```python
from build123d import *

# Parameters (mm, degrees)
EXTRUDE_1_DEPTH = 3
FILLET_1_R      = 1.5


with BuildPart() as part:
    # 草图1 → 凸台-拉伸1 (new body)
    with BuildSketch(Plane.XY):
        with BuildLine():
            Line((100.55, -9.975), (100.55, 9.975))
            Line((100.55, 9.975), (93.45, 9.975))
            ThreePointArc((93.45, 9.975), (92.4, 11.025), (93.45, 12.075))
            Line((93.45, 12.075), (93.45, 14.975))
            Line((93.45, 14.975), (49.05, 14.975))
            Line((49.05, 14.975), (49.05, 12.125))
            ThreePointArc((49.05, 12.125), (49.79246212, 11.81746212), (50.1, 11.075))
            ThreePointArc((50.1, 11.075), (49.79246212, 10.33253788), (49.05, 10.025))
            Line((49.05, 10.025), (45.95, 10.025))
            ThreePointArc((45.95, 10.025), (44.9, 11.075), (45.95, 12.125))
            Line((45.95, 12.125), (45.95, 14.975))
            Line((45.95, 14.975), (1.55, 14.975))
            Line((1.55, 14.975), (1.55, 12.075))
            ThreePointArc((1.55, 12.075), (2.29246212, 11.76746212), (2.6, 11.025))
            ThreePointArc((2.6, 11.025), (2.29246212, 10.28253788), (1.55, 9.975))
            Line((1.55, 9.975), (-5.55, 9.975))
            Line((-5.55, 9.975), (-5.55, -9.975))
            Line((-5.55, -9.975), (1.55, -9.975))
            ThreePointArc((1.55, -9.975), (2.29246212, -10.28253788), (2.6, -11.025))
            ThreePointArc((2.6, -11.025), (2.29246212, -11.76746212), (1.55, -12.075))
            Line((1.55, -12.075), (1.55, -14.975))
            Line((1.55, -14.975), (45.95, -14.975))
            Line((45.95, -14.975), (45.95, -12.125))
            ThreePointArc((45.95, -12.125), (44.9, -11.075), (45.95, -10.025))
            Line((45.95, -10.025), (49.05, -10.025))
            ThreePointArc((49.05, -10.025), (49.79246212, -10.33253788), (50.1, -11.075))
            ThreePointArc((50.1, -11.075), (49.79246212, -11.81746212), (49.05, -12.125))
            Line((49.05, -12.125), (49.05, -14.975))
            Line((49.05, -14.975), (93.45, -14.975))
            Line((93.45, -14.975), (93.45, -12.075))
            ThreePointArc((93.45, -12.075), (92.4, -11.025), (93.45, -9.975))
            Line((93.45, -9.975), (100.55, -9.975))
        make_face()
        with BuildLine():
            ThreePointArc((2.6, -3.075), (2.29246212, -3.81746212), (1.55, -4.125))
            Line((1.55, -4.125), (-1.55, -4.125))
            ThreePointArc((-1.55, -4.125), (-2.6, -3.075), (-1.55, -2.025))
            Line((-1.55, -2.025), (-1.55, 2.025))
            ThreePointArc((-1.55, 2.025), (-2.6, 3.075), (-1.55, 4.125))
            Line((-1.55, 4.125), (1.55, 4.125))
            ThreePointArc((1.55, 4.125), (2.29246212, 3.81746212), (2.6, 3.075))
            ThreePointArc((2.6, 3.075), (2.29246212, 2.33253788), (1.55, 2.025))
            Line((1.55, 2.025), (1.55, -2.025))
            ThreePointArc((1.55, -2.025), (2.29246212, -2.33253788), (2.6, -3.075))
        make_face(mode=Mode.SUBTRACT)
        Polygon((39.221033587, -11.975), (8.278966413, -11.975), (23.75, -1.795569934), align=None, mode=Mode.SUBTRACT)
        Polygon((26.478966413, 0), (41.95, 10.179430066), (41.95, -10.179430066), align=None, mode=Mode.SUBTRACT)
        with BuildLine():
            ThreePointArc((50.1, -3.075), (49.79246212, -3.81746212), (49.05, -4.125))
            Line((49.05, -4.125), (45.95, -4.125))
            ThreePointArc((45.95, -4.125), (44.9, -3.075), (45.95, -2.025))
            Line((45.95, -2.025), (45.95, 2.025))
            ThreePointArc((45.95, 2.025), (44.9, 3.075), (45.95, 4.125))
            Line((45.95, 4.125), (49.05, 4.125))
            ThreePointArc((49.05, 4.125), (49.79246212, 3.81746212), (50.1, 3.075))
            ThreePointArc((50.1, 3.075), (49.79246212, 2.33253788), (49.05, 2.025))
            Line((49.05, 2.025), (49.05, -2.025))
            ThreePointArc((49.05, -2.025), (49.79246212, -2.33253788), (50.1, -3.075))
        make_face(mode=Mode.SUBTRACT)
        Polygon((55.778966413, -11.975), (71.25, -1.795569934), (86.721033587, -11.975), align=None, mode=Mode.SUBTRACT)
        Polygon((53.05, 10.179430066), (68.521033587, 0), (53.05, -10.179430066), align=None, mode=Mode.SUBTRACT)
        with BuildLine():
            ThreePointArc((97.6, -3.075), (97.29246212, -3.81746212), (96.55, -4.125))
            Line((96.55, -4.125), (93.45, -4.125))
            ThreePointArc((93.45, -4.125), (92.4, -3.075), (93.45, -2.025))
            Line((93.45, -2.025), (93.45, 2.025))
            ThreePointArc((93.45, 2.025), (92.4, 3.075), (93.45, 4.125))
            Line((93.45, 4.125), (96.55, 4.125))
            ThreePointArc((96.55, 4.125), (97.29246212, 3.81746212), (97.6, 3.075))
            ThreePointArc((97.6, 3.075), (97.29246212, 2.33253788), (96.55, 2.025))
            Line((96.55, 2.025), (96.55, -2.025))
            ThreePointArc((96.55, -2.025), (97.29246212, -2.33253788), (97.6, -3.075))
        make_face(mode=Mode.SUBTRACT)
        Polygon((21.021033587, 0), (5.55, -10.179430066), (5.55, 10.179430066), align=None, mode=Mode.SUBTRACT)
        Polygon((23.75, 1.795569934), (8.278966413, 11.975), (39.221033587, 11.975), align=None, mode=Mode.SUBTRACT)
        Polygon((55.778966413, 11.975), (86.721033587, 11.975), (71.25, 1.795569934), align=None, mode=Mode.SUBTRACT)
        Polygon((89.45, 10.179430066), (89.45, -10.179430066), (73.978966413, 0), align=None, mode=Mode.SUBTRACT)
    extrude(amount=EXTRUDE_1_DEPTH)

    # 圆角1
    fillet_1_edges = [part.edges().sort_by_distance(p)[0] for p in [
        (55.778966413, 11.975, 1.5),
        (71.25, 1.795569934, 1.5),
        (86.721033587, 11.975, 1.5),
        (8.278966413, -11.975, 1.5),
        (39.221033587, -11.975, 1.5),
        (23.75, -1.795569934, 1.5),
        (41.95, -10.179430066, 1.5),
        (41.95, 10.179430066, 1.5),
        (26.478966413, 0, 1.5),
        (21.021033587, 0, 1.5),
        (5.55, 10.179430066, 1.5),
        (5.55, -10.179430066, 1.5),
        (39.221033587, 11.975, 1.5),
        (8.278966413, 11.975, 1.5),
        (23.75, 1.795569934, 1.5),
        (53.05, -10.179430066, 1.5),
        (68.521033587, 0, 1.5),
        (53.05, 10.179430066, 1.5),
        (86.721033587, -11.975, 1.5),
        (71.25, -1.795569934, 1.5),
        (55.778966413, -11.975, 1.5),
        (73.978966413, 0, 1.5),
        (89.45, -10.179430066, 1.5),
        (89.45, 10.179430066, 1.5),
    ]]
    fillet(fillet_1_edges, radius=FILLET_1_R)


solid = part.part
```
Work out the finished part from the listing and answer in its coordinate system (mm). A direction names the side the tool comes from. Give positions to 0.01 mm unless a question says otherwise; leave off trailing zeros. Write each loop counter-clockwise with the first axis right and the second up, starting at its lowest first coordinate (ties: lowest second). Pieces come first, ordered by that corner, then holes. Notation, with made-up numbers: (-6.75, -35) -> (22.25, -35) arc R24 cw to (22.25, 4) -> close; hole circle Ø7 at (48, 20.5). An arc over 180 degrees is marked (long way). Write item = value, one per line.
Q1. For a pull along X with two mould halves and no side action, classify faces 3 (the flat face through (1.55, -14, 1)), 4 (the flat face through (71, -14.975, 1)), 5 (the cylindrical face through (83.14, -10.93, 1.52)), 6 (the cylindrical face through (27.71, -0.02, 1.52)) as pulls with the +X half, pulls with the -X half, needs draft (parallel to the pull), parting line crosses it, or undercut.
Computed values:
face_3 = pulls with the -X half
face_4 = needs draft
face_5 = undercut
face_6 = undercut
Q2. Consider line 1 along Y through (x, z) = (46, 1.55) (3 decimals); line 2 along Y through (x, z) = (22.5, 1) (3 decimals); line 3 along Y through (x, z) = (30, 2.95) (3 decimals). Determine where each line is inside the solid, lowest interval first.
Computed values:
line_1 = -10.025 to -4.125, 4.125 to 10.025
line_2 = -14.975 to -11.975, -2.618 to 2.618, 11.975 to 14.975
line_3 = -14.975 to -11.975, -5.908 to -2.317, 2.317 to 5.908, 11.975 to 14.975
Q3. A tool of negligible diameter and unlimited length cuts with its end or side. For faces 1 (the cylindrical face through (41.182, 8.706, 1.521)), 2 (the cylindrical face through (92.4, 11, 1.5)), from which of +Z, -Z, +X, -X, +Y, -Y can it reach the whole face along a straight path? Write none if from no direction.
Computed values:
face_1 = +Z, -Z
face_2 = +Z, -Z, +X
Q4. Section B-B on y = -6.5 is taken. Determine the outline of the cut face in (x, z).
Computed values:
outline = (-5.55, 0) -> (5.55, 0) -> (5.55, 3) -> (-5.55, 3) -> close; (11.14, 0) -> (16.6, 0) -> (16.6, 3) -> (11.14, 3) -> close; (30.9, 0) -> (36.36, 0) -> (36.36, 3) -> (30.9, 3) -> close; (41.95, 0) -> (53.05, 0) -> (53.05, 3) -> (41.95, 3) -> close; (58.64, 0) -> (64.1, 0) -> (64.1, 3) -> (58.64, 3) -> close; (78.4, 0) -> (83.86, 0) -> (83.86, 3) -> (78.4, 3) -> close; (89.45, 0) -> (100.55, 0) -> (100.55, 3) -> (89.45, 3) -> close
Q5. Section A-A on x = 10.5 is taken. Determine the outline of the cut face in (y, z) (1 decimal).
Computed values:
outline = (-15, 0) -> (-6.9, 0) -> (-6.9, 3) -> (-15, 3) -> close; (6.9, 0) -> (15, 0) -> (15, 3) -> (6.9, 3) -> close
Q6. Flat-ended cylindrical pins translate along their axes: pin 1 Ø8 at (x, y) = (12, 1.5) entering from -Z; pin 2 Ø0.9 at (y, z) = (14, 2) entering from +X; pin 3 Ø0.9 at (x, z) = (47.5, 2) entering from +Y (3 decimals). Find the tip coordinate at first contact, or state that the pin passes through.
Computed values:
pin_1 = 0
pin_2 = 93.45
pin_3 = 10.025
Q7. Section C-C on z = 0.7 is taken. State how many separate pieces and enclosed holes the cut face has, and give its area (3 significant figures).
Computed values:
separate_pieces = 1
enclosed_holes = 11
area = 1,690 mm^2
